Source: CAD feature listing. Evaluate the final solid. Frame: model axes, mm. Face numbers are marked on the shaded views. A direction names the side the tool comes from. Give positions to 0.01 mm unless a question says otherwise; leave off trailing zeros. Loops run counter-clockwise (first coordinate to the right, second up) from the corner with the lowest first, then second, coordinate; pieces in that order, holes last.
from build123d import *

# Parameters (mm, degrees)
SKETCH1_W               = 45
SKETCH1_H               = 20
BOSS_EXTRUDE1_DEPTH     = 30
BOSS_EXTRUDE1_2_DEPTH   = 30
CUT_EXTRUDE1_DEPTH      = 90
CUT_EXTRUDE1_DEPTH_BACK = 90
SKETCH2_R               = 18.91234553
SKETCH4_W               = 200
SKETCH4_H               = 20
BOSS_EXTRUDE2_DEPTH     = 5
FILLET1_R               = 10
SKETCH5_W               = 3
SKETCH5_H               = 13.263798278
BOSS_EXTRUDE3_DEPTH     = 10
CHAMFER1_SIZE           = 2.108112521
CHAMFER1_SIZE_2         = 15
BOSS_EXTRUDE4_DEPTH     = 2
FILLET2_R               = 5
CUT_EXTRUDE2_DEPTH      = 111.469562822


# Some blends are built 0.0001 mm under size
with BuildPart() as part:
    # Sketch1 → Boss-Extrude1 (new body)
    with BuildSketch(Plane(origin=(0, 0, 0), x_dir=(1, 0, 0), z_dir=(0, 1, 0))):
        with Locations((-77.5, 0)):
            Rectangle(SKETCH1_W, SKETCH1_H)
    extrude(amount=BOSS_EXTRUDE1_DEPTH)


with BuildPart() as body_2:
    # Sketch1 → Boss-Extrude1 2 (new body)
    with BuildSketch(Plane(origin=(0, 0, 0), x_dir=(1, 0, 0), z_dir=(0, 1, 0))):
        with Locations((77.5, 0)):
            Rectangle(SKETCH1_W, SKETCH1_H)
    extrude(amount=BOSS_EXTRUDE1_2_DEPTH)


with BuildPart() as cut_extrude1_tool:
    # Sketch2 → Cut-Extrude1 (new, two sides: drawn at the far end of the back side and taken through both)
    with BuildSketch(Plane(origin=(0, 0, 0), x_dir=(0, 0, -1), z_dir=(1, 0, 0)).offset(-CUT_EXTRUDE1_DEPTH_BACK)):
        with Locations((-21.83879207, 15)):
            Circle(SKETCH2_R)
    extrude(amount=CUT_EXTRUDE1_DEPTH + CUT_EXTRUDE1_DEPTH_BACK)


with BuildPart() as part_1:
    add(part.part)

    # Cut-Extrude1: cut by cut_extrude1_tool
    add(cut_extrude1_tool.part, mode=Mode.SUBTRACT)



with BuildPart() as body_2_1:
    add(body_2.part)

    # Cut-Extrude1: cut by cut_extrude1_tool
    add(cut_extrude1_tool.part, mode=Mode.SUBTRACT)


with BuildPart() as part_2:
    add(part_1.part)

    add(body_2_1.part)  # Boss-Extrude2 merges body 2
    # Sketch4 → Boss-Extrude2 (add)
    with BuildSketch(Plane(origin=(0, 30, 0), x_dir=(1, 0, 0), z_dir=(0, 1, 0))):
        Rectangle(SKETCH4_W, SKETCH4_H)
    extrude(amount=BOSS_EXTRUDE2_DEPTH)

    # Fillet1
    fillet1_edges = [part_2.edges().sort_by_distance(p)[0] for p in [
        (100, 17.5, 10),
        (-100, 35, 0),
        (100, 35, 0),
        (-100, 17.5, 10),
    ]]
    fillet(fillet1_edges, radius=FILLET1_R - 0.0001)  # a hair under: the kernel refuses the full size

    # Sketch5 → Boss-Extrude3 (add)
    with BuildSketch(Plane(origin=(0, 35, 0), x_dir=(1, 0, 0), z_dir=(0, 1, 0))):
        with Locations((-76.5, -0.54359829)):
            Rectangle(SKETCH5_W, SKETCH5_H)
        with Locations((76.5, -0.54359829)):
            Rectangle(SKETCH5_W, SKETCH5_H)
    extrude(amount=BOSS_EXTRUDE3_DEPTH)

    # Chamfer1
    # the kernel refuses this chamfer: 15, 2.108112521 mm, written as the material it takes off along each edge
    with BuildSketch(Plane(origin=(-116.985961034, 45, -6.088300849), x_dir=(0, -0.9651598825854408, -0.26166085119417143), z_dir=(1, 0, 0)), Plane(origin=(36.014038966, 45, -6.088300849), x_dir=(0, -0.9651598825854406, -0.26166085119417176), z_dir=(1, 0, 0))) as chamfer1_piece_1:
        Polygon((CHAMFER1_SIZE * 0.965159882373, -CHAMFER1_SIZE * 0.261660851137), (-CHAMFER1_SIZE_2 * 0.261660851194, -CHAMFER1_SIZE_2 * 0.965159882585), (0, 0), align=None)
    extrude(amount=80.971922068, mode=Mode.SUBTRACT)

    # Sketch6 → Boss-Extrude4 (add)
    with BuildSketch(Plane(origin=(0, 42.900189564, -6.02922845), x_dir=(1, 0, 0), z_dir=(0, 0.9902680687415693, -0.13917310096007307))):
        with BuildLine():
            Line((-98, 4.441058829), (-98, -31.70498546))
            ThreePointArc((-98, -31.70498546), (0.017055636, -22.045990643), (98, -32.045090114))
            Line((98, -32.045090114), (98, 3.690476172))
            ThreePointArc((98, 3.690476172), (0.081000585, 25.217488155), (-98, 4.441058829))
        make_face()
    extrude(amount=BOSS_EXTRUDE4_DEPTH)

    # Fillet2
    fillet2_edges = [part_2.edges().sort_by_distance(p)[0] for p in [
        (98, 43.37684262, -9.822962262),
        (-98, 43.272381704, -10.566240301),
        (-98, 48.302938775, 25.22803317),
        (98, 48.350272194, 25.564827949),
    ]]
    fillet(fillet2_edges, radius=FILLET2_R)

    # Sketch7 → Cut-Extrude2 (cut, through all)
    with BuildSketch(Plane(origin=(0, 35, 0), x_dir=(1, 0, 0), z_dir=(0, 1, 0))):
        Polygon((-40, -10), (-35, -2.397862122), (35, -2.397862122), (40, -10), align=None)
    extrude(amount=-CUT_EXTRUDE2_DEPTH, mode=Mode.SUBTRACT)


solid = part_2.part
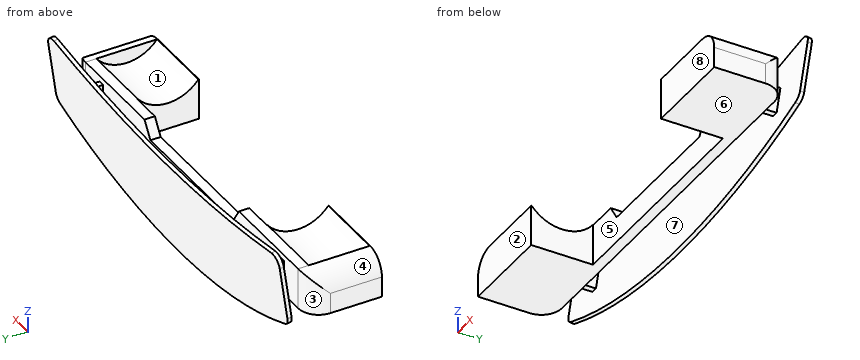
1) Pull-direction query (Y, two-part tool) for the marked faces 6, 7 and 8; classes: released by +Y, released by -Y, zero draft, split by the parting line, or undercut.
Checks:
face 6: zero draft
face 7: undercut
face 8: released by -Y
2) Cut plane C-C (z = -4). Return loops of the section in (x, y).
Checks:
outline: (-100, 0) - (-55, 0) - (-55, 30) - (55, 30) - (55, 0) - (100, 0) - (100, 25) arc R10 ccw to (90, 35) - (78, 35) - (78, 43.19) - (98, 43.19) - (98, 45.21) - (-98, 45.21) - (-98, 43.19) - (-78, 43.19) - (-78, 35) - (-90, 35) arc R10 ccw to (-100, 25) - close; hole (-75, 35) - (75, 35) - (75, 43.19) - (-75, 43.19) - close
3) Cut plane D-D (y = 32). Return loops of the section in (x, z), and give its area (3 significant figures).
Checks:
outline: (-97.14, -10) - (97.14, -10) - (97.14, 7) arc R10 ccw to (90, 10) - (40, 10) - (35, 2.4) - (-35, 2.4) - (-40, 10) - (-90, 10) arc R10 ccw to (-97.14, 7) - close
area: 3,300 mm2
4) Reachability of the marked faces 1, 2, 3, 4 and 5 from +Z, -Z, +X, -X, +Y, -Y: full face, straight path, thin tool, end or side. Return the list, or none.
Checks:
face 1: +Z
face 2: +Z, -Z, +X, -X, -Y
face 3: +Z, -Z, -X
face 4: +Z, -X, -Y
face 5: +Z, -Z, -Y
5) Ray query, probe 1 along Y at (x, z) = (52, -7.5); probe 2 along X at (y, z) = (36, 1.5); probe 3 along X at (y, z) = (17.5, -8). Return the intervals inside material, ascending.
Checks:
probe 1: y = 30 to 35, 42.69 to 44.71
probe 2: x = -78 to -75, 75 to 78
probe 3: x = -100 to -55, 55 to 100
6) Contact query for flat-ended pins moving along their axis: P1, Ø17.5, axis at x = 61, y = 17, coming from the +Z side; P2, Ø5, axis at y = 42, z = 1, coming from the -X side; P3, Ø4, axis at x = -10, z = -6, coming from the -Y side. Output: stop coordinate, or through.
Checks:
P1: stops at z = 6.28
P2: stops at x = -98
P3: stops at y = 30
7) Cut plane B-B (x = -5). Return loops of the section in (y, z).
Checks:
outline: (30, -10) - (35, -10) - (35, 2.4) - (30, 2.4) - close; (39.4, -30.97) - (41.38, -31.25) - (47.95, 15.54) - (45.97, 15.82) - close
